Here's how the part is built. I have some questions about the finished solid (model axes, mm). A direction names the side the tool comes from. Round coordinates to 2 decimals unless told otherwise and drop trailing zeros. Loops run counter-clockwise (first coordinate to the right, second up) from the corner with the lowest first, then second, coordinate; pieces in that order, holes last. Notation, with made-up numbers: (37.5, 13.25) -> (94.5, 13.25) arc R16 cw to (94.5, 38.25) -> close; hole circle Ø4 at (-29.5, 80.25). An arc over 180 degrees is marked (long way). Use CSV: the item, a comma, the result in double quotes. Start each with the question number.
from build123d import *

# Parameters (mm, degrees)
F0_W     = 70
F0_H     = 130
F1_DEPTH = 60
F2_R     = 2
F3_W     = 64
F3_H     = 124
F4_DEPTH = 56


with BuildPart() as f1:
    # F0 (on Top) → F1 (new body)
    with BuildSketch(Plane.XY):
        with Locations((-1.721807, 8.950054)):
            Rectangle(F0_W, F0_H)
    extrude(amount=F1_DEPTH)

    # F2
    f2_edges = [f1.edges().sort_by_distance(p)[0] for p in [
        (33.278193, 73.950054, 30),
        (33.278193, -56.049946, 30),
        (-36.721807, 73.950054, 30),
        (-36.721807, -56.049946, 30),
    ]]
    fillet(f2_edges, radius=F2_R)

    # F3 (on face) → F4 (cut)
    with BuildSketch(Plane.XY.offset(60)):
        with Locations((-1.721807, 8.950054)):
            Rectangle(F3_W, F3_H)
    extrude(amount=-F4_DEPTH, mode=Mode.SUBTRACT)


solid = f1.part
Q1. Will this pin go through, and if not, where does the flat tip stop? pin 1 Ø1.5 at (x, y) = (-16.5, 8.5) entering from +Z.
Q2. I need wall thicknesses on line 1 along Y through (x, z) = (-6.5, 56); line 2 along X through (y, z) = (68.5, 50.5); line 3 along Z through (x, y) = (-31.5, 15). Which ranges of each line are inside material? Lowest first, please.
Q3. I want a section at C-C, the plane y = -14.5. List the corners of the cut face in (x, z) for me.
Q4. I want a section at A-A, the plane z = 15.5. List the corners of the cut face in (x, y) for me.
Q5. I want a section at B-B, the plane x = -26.5. List the corners of the cut face in (y, z) for me.
Q6. If we mould it in two halves opening along X, with no side actions, what happens to faces 3 (the flat face through (-2, 73.95, 30)), 4 (the flat face through (-33.722, 8, 32)), 5 (the flat face through (-36.722, 8, 30))? For each: pulls with the +X half, pulls with the -X half, needs draft (parallel to the pull), parting line crosses it, or undercut.
Q7. For faces 1 (the flat face through (-2, -56.05, 30)), 2 (the flat face through (-2, 70.95, 32)), which set-ups out of +Z, -Z, +X, -X, +Y, -Y let a thin tool reach every point of the face, with its end or its side?
Values found:
1,pin 1,"z = 4"
2,line 1,"-56.05 to -53.05, 70.95 to 73.95"
2,line 2,"-36.72 to -33.72, 30.28 to 33.28"
2,line 3,"0 to 4"
3,outline,"(-36.72, 0) -> (33.28, 0) -> (33.28, 60) -> (30.28, 60) -> (30.28, 4) -> (-33.72, 4) -> (-33.72, 60) -> (-36.72, 60) -> close"
4,outline,"(-36.72, -54.05) arc R2 ccw to (-34.72, -56.05) -> (31.28, -56.05) arc R2 ccw to (33.28, -54.05) -> (33.28, 71.95) arc R2 ccw to (31.28, 73.95) -> (-34.72, 73.95) arc R2 ccw to (-36.72, 71.95) -> close; hole (-33.72, -53.05) -> (30.28, -53.05) -> (30.28, 70.95) -> (-33.72, 70.95) -> close"
5,outline,"(-56.05, 0) -> (73.95, 0) -> (73.95, 60) -> (70.95, 60) -> (70.95, 4) -> (-53.05, 4) -> (-53.05, 60) -> (-56.05, 60) -> close"
6,face 3,"needs draft"
6,face 4,"undercut"
6,face 5,"pulls with the -X half"
7,face 1,"+Z, -Z, +X, -X, -Y"
7,face 2,"+Z"
